Source: CAD feature listing. Evaluate the final solid. Frame: model axes, mm. A direction names the side the tool comes from. Coordinates: 2 decimals unless noted, no trailing zeros. Loops run counter-clockwise (first coordinate to the right, second up) from the corner with the lowest first, then second, coordinate; pieces in that order, holes last.
Item 1: Pull-direction query (X, two-part tool) for faces 1 (the cylindrical face through (12.9, -1.2, 62.1)), 2 (the cylindrical face through (21.27, 6.7, 33.03)), 3 (the flat face through (0, -5, 0)); classes: +X half, -X half, draft (parallel to the pull), parting line (faces both ways), or undercut.
Item 2: Section query D-D, the plane x = -6. Return the cut outline in (y, z), then the cut area to 3 significant figures.
Item 3: Section query A-A, the plane x = 0. Return the cut outline in (y, z).
Item 4: Reachability of faces 4 (the flat face through (0, 0, 113)), 5 (the cylindrical face through (-2.5, -0.1, -3.5)), 6 (the flat face through (0, -10, 67)) from +Z, -Z, +X, -X, +Y, -Y: full face, straight path, thin tool, end or side. Return the list, or none.
Item 5: Pin query (flat end, axial travel): pin 1 Ø1.5 at (y, z) = (1, 34) entering from +X; pin 2 Ø6 at (x, y) = (13.5, 9.5) entering from -Z; pin 3 Ø3 at (x, z) = (-17, 49.5) entering from -Y; pin 4 Ø10 at (x, z) = (16.5, 101) entering from +Y. Return the tip coordinate at first contact, or that it passes through.
Item 6: Section query B-B, the plane y = 0. Return the cut outline in (x, z), then the cut area to 3 significant figures.
Item 7: Line query: probe 1 along Z at (x, y) = (-0.5, 4.5); probe 2 along Z at (x, y) = (-7, 6); probe 3 along Y at (x, z) = (-14, 60). Output: solid intervals per line, ascending.
Item 8: Section query C-C, the plane z = 64.5. Return the cut outline in (x, y), then the cut area to 3 significant figures.
```python
from build123d import *

# Parameters (mm, degrees)
SKETCH_1_R          = 22.3
EXTRUDE_1_DEPTH     = 67
SKETCH_2_R          = 8.5
EXTRUDE_2_DEPTH     = 46
SKETCH_3_R          = 2.5
EXTRUDE_3_DEPTH     = 7
SKETCH_4_R          = 2
CUT_EXTRUDE_1_DEPTH = 10


with BuildPart() as part:
    # 草圖1 → 填料-伸長1 (new body)
    with BuildSketch(Plane.XY):
        Circle(SKETCH_1_R)
    extrude(amount=EXTRUDE_1_DEPTH)

    # 草圖2 → 填料-伸長2 (add)
    with BuildSketch(Plane.XY.offset(67)):
        Circle(SKETCH_2_R)
    extrude(amount=EXTRUDE_2_DEPTH)

    # 草圖3 → 填料-伸長3 (add)
    with BuildSketch(Plane(origin=(0, 0, 0), x_dir=(-1, 0, 0), z_dir=(0, 0, -1))):
        with Locations(Location((0, 0, 0), (0, 0, 180))):
            Circle(SKETCH_3_R)
    extrude(amount=EXTRUDE_3_DEPTH)

    # 草圖4 → 除料-伸長1 (cut)
    with BuildSketch(Plane.XY.offset(67)):
        with Locations((14.5, 0)):
            Circle(SKETCH_4_R)
        with Locations(Location((-14.5, 0, 0), (0, 0, 180))):
            Circle(SKETCH_4_R)
    extrude(amount=-CUT_EXTRUDE_1_DEPTH, mode=Mode.SUBTRACT)


solid = part.part
```
Verdict:
1. face 1: undercut
1. face 2: parting line
1. face 3: draft
2. outline: (-21.48, 0) - (21.48, 0) - (21.48, 67) - (6.02, 67) - (6.02, 113) - (-6.02, 113) - (-6.02, 67) - (-21.48, 67) - close
2. area: 3,430 mm2
3. outline: (-22.3, 0) - (-2.5, 0) - (-2.5, -7) - (2.5, -7) - (2.5, 0) - (22.3, 0) - (22.3, 67) - (8.5, 67) - (8.5, 113) - (-8.5, 113) - (-8.5, 67) - (-22.3, 67) - close
4. face 4: +Z, +X, -X, +Y, -Y
4. face 5: -Z
4. face 6: +Z
5. pin 1: stops at x = 22.3
5. pin 2: stops at z = 0
5. pin 3: stops at y = -16.03
5. pin 4: passes through
6. outline: (-22.3, 0) - (-2.5, 0) - (-2.5, -7) - (2.5, -7) - (2.5, 0) - (22.3, 0) - (22.3, 67) - (16.5, 67) - (16.5, 57) - (12.5, 57) - (12.5, 67) - (8.5, 67) - (8.5, 113) - (-8.5, 113) - (-8.5, 67) - (-12.5, 67) - (-12.5, 57) - (-16.5, 57) - (-16.5, 67) - (-22.3, 67) - close
6. area: 3,730 mm2
7. probe 1: z = 0 to 113
7. probe 2: z = 0 to 67
7. probe 3: y = -17.36 to -1.94, 1.94 to 17.36
8. outline: circle Ø44.6 at (0, 0); hole circle Ø4 at (-14.5, 0); hole circle Ø4 at (14.5, 0)
8. area: 1,540 mm2
